Source: CAD feature listing. Evaluate the final solid. Frame: model axes, mm. Face numbers are marked on the shaded views. A direction names the side the tool comes from. Give positions to 0.01 mm unless a question says otherwise; leave off trailing zeros. Write each loop counter-clockwise with the first axis right and the second up, starting at its lowest first coordinate (ties: lowest second). Pieces come first, ordered by that corner, then holes. Notation, with made-up numbers: (68.5, 36) -> (83.5, 36) arc R23 cw to (83.5, 50) -> close; hole circle Ø4 at (-37, 34.5). An arc over 180 degrees is marked (long way). Write item = value, one per line.
from build123d import *

# Parameters (mm, degrees)
BOSS_EXTRUDE3_DEPTH      = 30
CHAMFER3_SIZE            = 2
CHAMFER4_SIZE            = 3
SKETCH5_R                = 40
CUT_EXTRUDE1_DEPTH       = 10
CHAMFER5_SIZE            = 1
SKETCH8_W                = 101.820371212
SKETCH8_H                = 22.171572876
CUT_EXTRUDE5_DEPTH       = 3
SKETCH9_W                = 3
SKETCH9_H                = 25
CUT_EXTRUDE7_DEPTH       = 5
SKETCH11_W               = 101.820371212
SKETCH11_H               = 22.171572876
CUT_EXTRUDE9_DEPTH       = 3
SKETCH12_R               = 41
CUT_EXTRUDE13_DEPTH      = 10
CUT_EXTRUDE13_DEPTH_BACK = 10
CHAMFER7_SIZE            = 1
SKETCH13_R               = 1.6
CUT_EXTRUDE14_DEPTH      = 20
SKETCH14_R               = 1.6
CUT_EXTRUDE15_DEPTH      = 20
SKETCH18_OUTSIDE_W       = 178.11
SKETCH18_OUTSIDE_H       = 148.11
SKETCH18_OUTSIDE_R       = 60
CUT_EXTRUDE16_DEPTH      = 60
BOSS_EXTRUDE6_DEPTH      = 1
SKETCH21_W               = 10
SKETCH21_H               = 10
CUT_EXTRUDE20_DEPTH      = 5
SKETCH24_R               = 2.5
CUT_EXTRUDE22_DEPTH      = 12


with BuildPart() as part:
    # Sketch2 → Boss-Extrude3 (new body)
    with BuildSketch(Plane(origin=(0, 0, 0), x_dir=(1, 0, 0), z_dir=(0, 1, 0))):
        Polygon((52.324399168, 55), (70, 40.283576004), (70, -40.283576004), (52.324399168, -55), (-52.324399168, -55), (-70, -40.283576004), (-70, 40.283576004), (-52.324399168, 55), align=None)
    extrude(amount=BOSS_EXTRUDE3_DEPTH)

    # Chamfer3
    chamfer3_edges = [part.edges().sort_by_distance(p)[0] for p in [
        (0, 30, 55),
        (61.162199584, 30, 47.641788002),
        (70, 30, 0),
        (61.162199584, 30, -47.641788002),
        (0, 30, -55),
        (-61.162199584, 30, -47.641788002),
        (-70, 30, 0),
        (-61.162199584, 30, 47.641788002),
    ]]
    chamfer(chamfer3_edges, length=CHAMFER3_SIZE)

    # Chamfer4
    chamfer4_edges = [part.edges().sort_by_distance(p)[0] for p in [
        (61.162199584, 0, 47.641788002),
        (0, 0, 55),
        (-61.162199584, 0, 47.641788002),
        (-70, 0, 0),
        (-61.162199584, 0, -47.641788002),
        (0, 0, -55),
        (61.162199584, 0, -47.641788002),
        (70, 0, 0),
    ]]
    chamfer(chamfer4_edges, length=CHAMFER4_SIZE)

    # Sketch5 → Cut-Extrude1 (cut)
    with BuildSketch(Plane.XZ):
        Circle(SKETCH5_R)
    extrude(amount=-CUT_EXTRUDE1_DEPTH, mode=Mode.SUBTRACT)

    # Chamfer5
    chamfer5_edges = [part.edges().sort_by_distance(p)[0] for p in [
        (-40, 0, 0),
    ]]
    chamfer(chamfer5_edges, length=CHAMFER5_SIZE)

    # Sketch8 → Cut-Extrude5 (cut)
    with BuildSketch(Plane.XY.offset(55)):
        with Locations((0, 15.5)):
            Rectangle(SKETCH8_W, SKETCH8_H)
    extrude(amount=-CUT_EXTRUDE5_DEPTH, mode=Mode.SUBTRACT)

    # Sketch9 → Cut-Extrude7 (cut)
    with BuildSketch(Plane.XZ):
        with BuildLine():
            Line((67, 12.5), (39.048047326, 12.5))
            ThreePointArc((39.048047326, 12.5), (40.50907269, 6.32574342), (41, 0))
            ThreePointArc((41, 0), (40.50907269, -6.32574342), (39.048047326, -12.5))
            Line((39.048047326, -12.5), (67, -12.5))
            Line((67, -12.5), (67, 12.5))
        make_face()
        with Locations((68.5, 0)):
            Rectangle(SKETCH9_W, SKETCH9_H)
        with BuildLine():
            Line((39.048047326, 12.5), (37.996710384, 12.5))
            ThreePointArc((37.996710384, 12.5), (40, 0), (37.996710384, -12.5))
            Line((37.996710384, -12.5), (39.048047326, -12.5))
            ThreePointArc((39.048047326, -12.5), (40.50907269, -6.32574342), (41, 0))
            ThreePointArc((41, 0), (40.50907269, 6.32574342), (39.048047326, 12.5))
        make_face()
        with BuildLine():
            Line((-37.996710384, 12.5), (-70, 12.5))
            Line((-70, 12.5), (-70, -12.5))
            Line((-70, -12.5), (-37.996710384, -12.5))
            ThreePointArc((-37.996710384, -12.5), (-40, 0), (-37.996710384, 12.5))
        make_face()
    extrude(amount=-CUT_EXTRUDE7_DEPTH, mode=Mode.SUBTRACT)

    # Sketch11 → Cut-Extrude9 (cut)
    with BuildSketch(Plane(origin=(0, 0, -55), x_dir=(-1, 0, 0), z_dir=(0, 0, -1))):
        with Locations((0, 15.5)):
            Rectangle(SKETCH11_W, SKETCH11_H)
    extrude(amount=-CUT_EXTRUDE9_DEPTH, mode=Mode.SUBTRACT)

    # Sketch12 → Cut-Extrude13 (cut, two sides)
    with BuildSketch(Plane.XZ.offset(-10)) as cut_extrude13_sk:
        Circle(SKETCH12_R)
    extrude(amount=CUT_EXTRUDE13_DEPTH, mode=Mode.SUBTRACT)
    extrude(cut_extrude13_sk.sketch, amount=-CUT_EXTRUDE13_DEPTH_BACK, mode=Mode.SUBTRACT)

    # Chamfer7
    chamfer7_edges = [part.edges().sort_by_distance(p)[0] for p in [
        (0, 0, -41),
    ]]
    chamfer(chamfer7_edges, length=CHAMFER7_SIZE)

    # Sketch13 → Cut-Extrude14 (cut)
    with BuildSketch(Plane.XZ.offset(-20)):
        with Locations((0, 14)):
            Circle(SKETCH13_R)
        with Locations((12.124355653, -7)):
            Circle(SKETCH13_R)
        with Locations((-12.124355653, -7)):
            Circle(SKETCH13_R)
    extrude(amount=-CUT_EXTRUDE14_DEPTH, mode=Mode.SUBTRACT)

    # Sketch14 → Cut-Extrude15 (cut)
    with BuildSketch(Plane.XZ.offset(-20)):
        with Locations((0, 34)):
            Circle(SKETCH14_R)
        with Locations((29.444863729, 17)):
            Circle(SKETCH14_R)
        with Locations((29.444863729, -17)):
            Circle(SKETCH14_R)
        with Locations((0, -34)):
            Circle(SKETCH14_R)
        with Locations((-29.444863729, -17)):
            Circle(SKETCH14_R)
        with Locations((-29.444863729, 17)):
            Circle(SKETCH14_R)
    extrude(amount=-CUT_EXTRUDE15_DEPTH, mode=Mode.SUBTRACT)

    # Sketch18 outside → Cut-Extrude16 (cut)
    with BuildSketch(Plane(origin=(0, 30, 0), x_dir=(1, 0, 0), z_dir=(0, 1, 0))):
        Rectangle(SKETCH18_OUTSIDE_W, SKETCH18_OUTSIDE_H)
        Circle(SKETCH18_OUTSIDE_R, mode=Mode.SUBTRACT)
    extrude(amount=-CUT_EXTRUDE16_DEPTH, mode=Mode.SUBTRACT)

    # Sketch19 → Boss-Extrude6 (add)
    with BuildSketch(Plane.XY.offset(52)):
        Polygon((-15.576923077, 20.5), (-14.679487179, 20.5), (-14.679487179, 11.525641026), (-10.833333333, 11.525641026), (-10.833333333, 10.5), (-15.576923077, 10.5), align=None)
        Polygon((-9.935897436, 20.5), (-8.908253205, 20.5), (-6.280048077, 16.203125), (-3.655849359, 20.5), (-2.628205128, 20.5), (-5.833333333, 15.253605769), (-5.833333333, 10.5), (-6.730769231, 10.5), (-6.730769231, 15.253605769), align=None)
        with BuildLine():
            Line((-0.833333333, 20.5), (1.16786859, 20.5))
            add(Edge.make_bspline(
                [(1.16786859, 20.5), (1.301414671, 20.499555469), (1.557837941, 20.498701919), (1.925190142, 20.493942596), (2.258981848, 20.48030158), (2.559038531, 20.46856277), (2.825354689, 20.447157224), (3.058746948, 20.426698232), (3.258140369, 20.399916344), (3.378842802, 20.375043707), (3.43349359, 20.363782051)],
                knots=[0, 0, 0, 0, 0.000400646, 0.000769285, 0.001102034, 0.001402842, 0.00167002, 0.001903434, 0.002105708, 0.002273069, 0.002273069, 0.002273069, 0.002273069], degree=3))
            add(Edge.make_bspline(
                [(3.43349359, 20.363782051), (3.506655373, 20.345705579), (3.6514182, 20.309938254), (3.85984696, 20.234339395), (4.058459314, 20.146854753), (4.246430241, 20.044101266), (4.422818216, 19.925316181), (4.589441961, 19.792550117), (4.747057571, 19.646529529), (4.8892908, 19.483572839), (5.023402376, 19.312611383), (5.136512737, 19.127743506), (5.234016965, 18.934424856), (5.311647014, 18.730689377), (5.374155509, 18.518512886), (5.418230479, 18.295973467), (5.444662444, 18.064084967), (5.447353459, 17.905919513), (5.448717949, 17.825721154)],
                knots=[0, 0, 0, 0, 0.000225945, 0.00044707, 0.000664092, 0.000876564, 0.0010888, 0.001301225, 0.001515231, 0.001732327, 0.001949488, 0.002166288, 0.002381294, 0.002598178, 0.002819412, 0.003044128, 0.003277954, 0.003518473, 0.003518473, 0.003518473, 0.003518473], degree=3))
            add(Edge.make_bspline(
                [(5.448717949, 17.825721154), (5.444520811, 17.692477998), (5.436331109, 17.43248609), (5.35997367, 17.055169286), (5.234897899, 16.703199815), (5.062545645, 16.37702085), (4.843061429, 16.082990434), (4.579276311, 15.824731991), (4.271043136, 15.608617955), (3.984102233, 15.458752798), (3.730633091, 15.362773059), (3.521966483, 15.295240606), (3.294346547, 15.243063562), (3.049954163, 15.196320328), (2.78777229, 15.161029773), (2.50842932, 15.13518236), (2.21172603, 15.119027935), (2.007900117, 15.116622207), (1.903044872, 15.115384615)],
                knots=[0, 0, 0, 0, 0.000399362, 0.000779259, 0.001149283, 0.001516695, 0.00188168, 0.00224574, 0.002619261, 0.003007206, 0.003213302, 0.003431872, 0.003664606, 0.003913302, 0.004178188, 0.004457849, 0.004754756, 0.005069316, 0.005069316, 0.005069316, 0.005069316], degree=3))
            Line((1.903044872, 15.115384615), (5.576923077, 10.5))
            Line((5.576923077, 10.5), (4.467147436, 10.5))
            Line((4.467147436, 10.5), (0.793269231, 15.115384615))
            Line((0.793269231, 15.115384615), (0.064102564, 15.115384615))
            Line((0.064102564, 15.115384615), (0.064102564, 10.5))
            Line((0.064102564, 10.5), (-0.833333333, 10.5))
            Line((-0.833333333, 10.5), (-0.833333333, 20.5))
        make_face()
        with BuildLine():
            Line((0.064102564, 19.474358974), (0.064102564, 16.141025641))
            Line((0.064102564, 16.141025641), (1.895032051, 16.127003205))
            add(Edge.make_bspline(
                [(1.895032051, 16.127003205), (1.980517877, 16.126965386), (2.146213754, 16.126892082), (2.385929939, 16.138302871), (2.609130259, 16.151283781), (2.814960979, 16.171139054), (3.003514051, 16.19672783), (3.174695232, 16.228736356), (3.328783952, 16.266027964), (3.508494061, 16.323746895), (3.709169865, 16.415192661), (3.927259751, 16.548236943), (4.112980716, 16.715577284), (4.269888894, 16.906930015), (4.395972984, 17.117319298), (4.484864567, 17.34422321), (4.541271545, 17.58191349), (4.547924532, 17.745279512), (4.551282051, 17.827724359)],
                knots=[0, 0, 0, 0, 0.000256418, 0.000497011, 0.000719809, 0.000927109, 0.001117203, 0.001290465, 0.001449339, 0.001592508, 0.00185611, 0.002109007, 0.002355881, 0.002602112, 0.002849125, 0.003088313, 0.0033308, 0.003577853, 0.003577853, 0.003577853, 0.003577853], degree=3))
            add(Edge.make_bspline(
                [(4.551282051, 17.827724359), (4.54784742, 17.908143141), (4.541041233, 18.067503823), (4.485473323, 18.300806424), (4.391503662, 18.52099771), (4.264868696, 18.727181953), (4.110585396, 18.914341198), (3.92967736, 19.074475921), (3.727091088, 19.206617249), (3.537744807, 19.291058336), (3.3685042, 19.342829345), (3.221562314, 19.379261242), (3.055529521, 19.408531153), (2.869599639, 19.431982755), (2.664566408, 19.452139739), (2.439393119, 19.46571625), (2.195573747, 19.473755861), (2.026582515, 19.474153258), (1.939102564, 19.474358974)],
                knots=[0, 0, 0, 0, 0.00024106, 0.000477692, 0.000714689, 0.000956555, 0.001201242, 0.001439631, 0.001678551, 0.001924252, 0.002058571, 0.002209185, 0.002378145, 0.002564001, 0.002771301, 0.002996098, 0.00324062, 0.003503048, 0.003503048, 0.003503048, 0.003503048], degree=3))
            Line((1.939102564, 19.474358974), (0.064102564, 19.474358974))
        make_face(mode=Mode.SUBTRACT)
        Polygon((11.730769231, 20.5), (16.346153846, 10.5), (15.370592949, 10.5), (13.892227564, 13.705128205), (9.358974359, 13.705128205), (7.838541667, 10.5), (6.858974359, 10.5), (11.602564103, 20.5), align=None)
        Polygon((11.656650641, 18.55088141), (9.845753205, 14.730769231), (13.419471154, 14.730769231), align=None, mode=Mode.SUBTRACT)
    extrude(amount=BOSS_EXTRUDE6_DEPTH)

    # Sketch21 → Cut-Extrude20 (cut)
    with BuildSketch(Plane(origin=(0, 30, 0), x_dir=(1, 0, 0), z_dir=(0, 1, 0))):
        with Locations((45, 17.5)):
            Rectangle(SKETCH21_W, SKETCH21_H)
        with Locations((-45, -17.5)):
            Rectangle(SKETCH21_W, SKETCH21_H)
        with Locations((-45, 17.5)):
            Rectangle(SKETCH21_W, SKETCH21_H)
        with Locations((45, -17.5)):
            Rectangle(SKETCH21_W, SKETCH21_H)
    extrude(amount=-CUT_EXTRUDE20_DEPTH, mode=Mode.SUBTRACT)

    # Sketch24 → Cut-Extrude22 (cut)
    with BuildSketch(Plane(origin=(0, 30, 0), x_dir=(1, 0, 0), z_dir=(0, 1, 0))):
        with Locations((-45, 17.5)):
            Circle(SKETCH24_R)
        with Locations((45, 17.5)):
            Circle(SKETCH24_R)
        with Locations((45, -17.5)):
            Circle(SKETCH24_R)
        with Locations((-45, -17.5)):
            Circle(SKETCH24_R)
    extrude(amount=-CUT_EXTRUDE22_DEPTH, mode=Mode.SUBTRACT)


solid = part.part
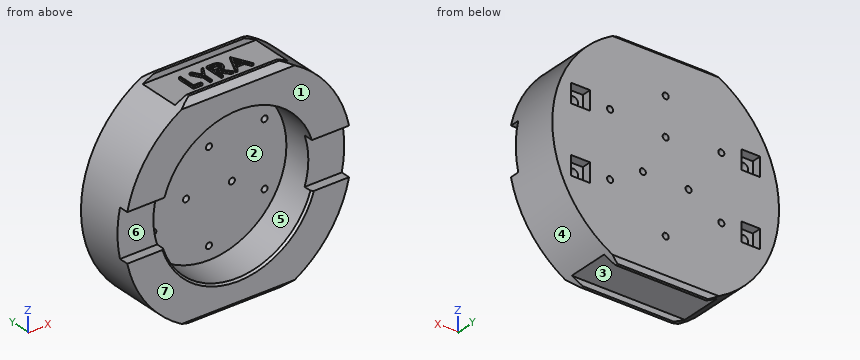
(1) Pull-direction query (Z, two-part tool) for the marked faces 1, 2, 3 and 4; classes: pulls with the +Z half, pulls with the -Z half, needs draft (parallel to the pull), parting line crosses it, or undercut.
Values follow:
face_1 = needs draft
face_2 = undercut
face_3 = pulls with the -Z half
face_4 = parting line crosses it
(2) Section query C-C (x = 44). Return loops of the section in (y, z).
Values follow:
outline = (0, -40.79) -> (30, -40.79) -> (30, -22.5) -> (25, -22.5) -> (25, -19.79) -> (18, -19.79) -> (18, -15.21) -> (25, -15.21) -> (25, -12.5) -> (30, -12.5) -> (30, 12.5) -> (25, 12.5) -> (25, 15.21) -> (18, 15.21) -> (18, 19.79) -> (25, 19.79) -> (25, 22.5) -> (30, 22.5) -> (30, 40.79) -> (0, 40.79) -> (0, 12.5) -> (5, 12.5) -> (5, -12.5) -> (0, -12.5) -> close
(3) Access query for the marked faces 5, 6 and 7. Directions: +Z, -Z, +X, -X, +Y, -Y. A direction counts if a zero-diameter tool reaches every point of the face in a straight line with its end or side. Return the directions, or none.
Values follow:
face_5 = -Y
face_6 = +X, -X, -Y
face_7 = +Z, -Z, +X, -X, -Y
(4) First-contact query: pin 1 (10 mm diameter, centred on y = 26.5, z = 23.5, fed in from +X); pin 2 (12 mm diameter, centred on x = 46, y = 7, fed in from +Z); pin 3 (4 mm diameter, centred on x = -12.12, z = -7, fed in from -Y). Flat tips, straight axial feed; report the tip coordinate or a pass-through.
Values follow:
pin_1 = 57.08
pin_2 = 44.72
pin_3 = 20
(5) Section query A-A (y = 7). Return loops of the section in (x, z), plus the area to 3 significant figures.
Values follow:
outline = (-29.93, -52) -> (29.93, -52) arc R60 ccw to (29.93, 52) -> (-29.93, 52) arc R60 ccw to start; hole circle Ø82 at (0, 0)
area = 5,380 mm2
(6) Section query B-B (z = 0). Return loops of the section in (x, y).
Values follow:
outline = (-60, 5) -> (-41, 5) -> (-41, 20) -> (41, 20) -> (41, 5) -> (60, 5) -> (60, 30) -> (-60, 30) -> close
(7) Section query D-D (z = 27). Return loops of the section in (x, y), plus the area to 3 significant figures.
Values follow:
outline = (-53.58, 0) -> (-30.85, 0) -> (-30.85, 20) -> (30.85, 20) -> (30.85, 0) -> (53.58, 0) -> (53.58, 30) -> (-53.58, 30) -> close
area = 1,980 mm2
(8) Material intervals for line 1 (Z direction, x = 0, y = 24.25); line 2 (Z direction, x = 0.5, y = 18); line 3 (Z direction, x = -45, y = 22.75), sorted ascending.
Values follow:
line_1 = -52 to -35.6, -32.4 to 12.4, 15.6 to 32.4, 35.6 to 52
line_2 = -52 to -41, 41 to 52
line_3 = -39.69 to -20, -15 to 15, 20 to 39.69
